Design review of the part shown in the three views and the two pictorial views. Dimensions are in mm from the part's minimum x, y and z. Round coordinates to 2 decimals unless told otherwise and drop trailing zeros. Write each loop counter-clockwise with the first axis right and the second up, starting at its lowest first coordinate (ties: lowest second). Pieces come first, ordered by that corner, then holes. Notation, with made-up numbers: (10, 66) -> (14, 66) arc R17 ccw to (14, 91) -> close; hole circle Ø2 at (-29.75, 76.5). An arc over 180 degrees is marked (long way). Return JSON: item names as keys, results as strings. Group by question number.
1. Clearance check with a flat-ended pin moving along its axis: P1, Ø6, axis at x = 22, y = 9, coming from the +Z side. State where the tip first meets the part, or that it passes through.
2. Take a section at A-A, the plane x = 22. Write out the cut boundary in (y, z).
3. Take a section at C-C, the plane y = 16.5. Write out the cut boundary in (x, z), then the cut area to 3 significant figures.
4. Take a section at B-B, the plane y = 2. Write out the cut boundary in (x, z).
5. Take a section at D-D, the plane x = 29. Write out the cut boundary in (y, z), then the cut area to 3 significant figures.
6. For line 1 along Z through (x, y) = (35.5, 17), list the stretches that pass through material, from the lowest coordinate up. Write a range as from..to.
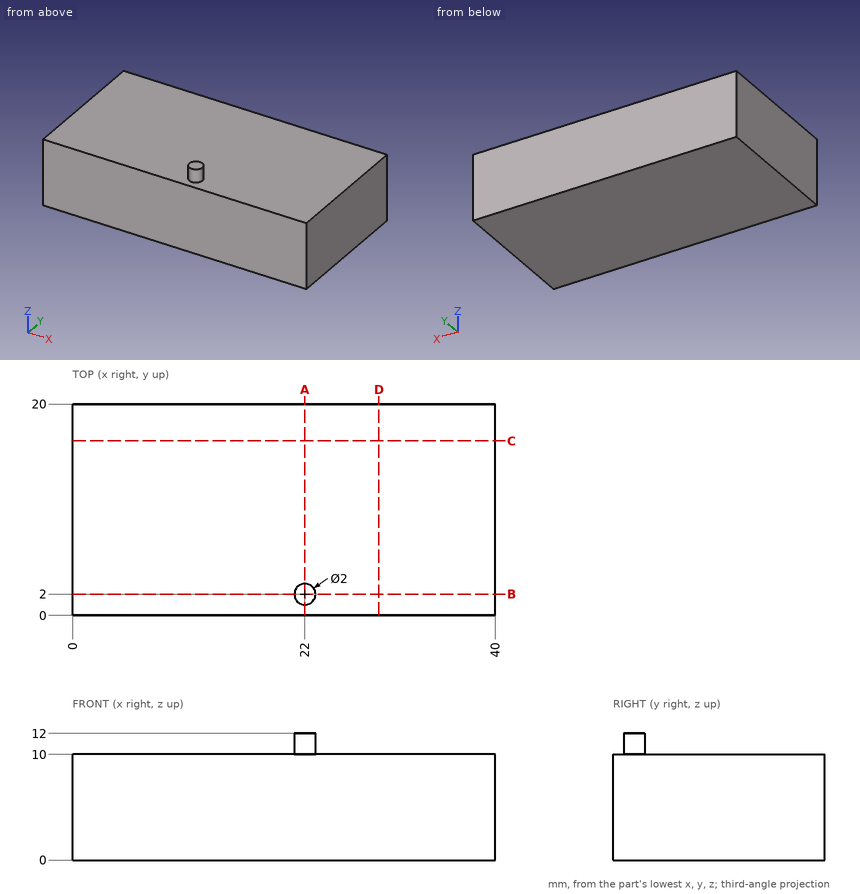
Output:
{
 "1": {"P1": "stops at z = 10"},
 "2": {"outline": "(0, 0) -> (20, 0) -> (20, 10) -> (3, 10) -> (3, 12) -> (1, 12) -> (1, 10) -> (0, 10) -> close"},
 "3": {"outline": "(0, 0) -> (40, 0) -> (40, 10) -> (0, 10) -> close", "area": "400 mm^2"},
 "4": {"outline": "(0, 0) -> (40, 0) -> (40, 10) -> (23, 10) -> (23, 12) -> (21, 12) -> (21, 10) -> (0, 10) -> close"},
 "5": {"outline": "(0, 0) -> (20, 0) -> (20, 10) -> (0, 10) -> close", "area": "200 mm^2"},
 "6": {"line 1": "z = 0..10"}
}
